from build123d import *

# Parameters (mm, degrees)
SKETCH1_R           = 25.4
BOSS_EXTRUDE1_DEPTH = 50
SKETCH2_W           = 8
SKETCH2_H           = 56.617696499
CUT_EXTRUDE1_DEPTH  = 30
SKETCH3_R           = 12.7
CUT_EXTRUDE2_DEPTH  = 35
SKETCH4_R           = 12.7
BOSS_EXTRUDE2_DEPTH = 50
BOSS_EXTRUDE3_START = -50
SKETCH5_R           = 12.7
BOSS_EXTRUDE3_DEPTH = 50


with BuildPart() as part:
    # Sketch1 → Boss-Extrude1 (new body)
    with BuildSketch(Plane.XY):
        Circle(SKETCH1_R)
    extrude(amount=BOSS_EXTRUDE1_DEPTH)

    # Sketch2 → Cut-Extrude1 (cut)
    with BuildSketch(Plane.XY.offset(50)):
        with Locations((0, -1.452503267)):
            Rectangle(SKETCH2_W, SKETCH2_H)
    extrude(amount=-CUT_EXTRUDE1_DEPTH, mode=Mode.SUBTRACT)

    # Sketch3 → Cut-Extrude2 (cut, symmetric)
    with BuildSketch(Plane.ZY.offset(-4)):
        with Locations(Location((31.954368174, 0, 0), (0, 0, 270))):
            Circle(SKETCH3_R)
    extrude(amount=CUT_EXTRUDE2_DEPTH, both=True, mode=Mode.SUBTRACT)

    # Mirror1: part across plane


with BuildPart() as part_1:
    add(part.part)
    add(part.part.mirror(Plane.XY))

    # Sketch4 → Boss-Extrude2 (add)
    with BuildSketch(Plane.ZY.offset(-4)):
        with Locations(Location((-32.054446032, 0, 0), (0, 0, 270))):
            Circle(SKETCH4_R)
    extrude(amount=-BOSS_EXTRUDE2_DEPTH)

    # Sketch5 → Boss-Extrude3 (add)
    with BuildSketch(Plane(origin=(-4, 0, 0), x_dir=(0, 0, -1), z_dir=(1, 0, 0)).offset(BOSS_EXTRUDE3_START)):
        with Locations(Location((32.054446032, 0, 0), (0, 0, 270))):
            Circle(SKETCH5_R)
    extrude(amount=BOSS_EXTRUDE3_DEPTH)


solid = part_1.part
Geometry: final body of the model. Coordinates: model frame, mm. A direction names the side the tool comes from. Round coordinates to 2 decimals unless told otherwise and drop trailing zeros. Loops run counter-clockwise (first coordinate to the right, second up) from the corner with the lowest first, then second, coordinate; pieces in that order, holes last. Notation, with made-up numbers: (69.5, 34.25) -> (84.5, 34.25) arc R11 cw to (84.5, 53.25) -> close; hole circle Ø8 at (42, -25). An arc over 180 degrees is marked (long way). One line per question, with ' | ' between items. Start each with the question number.
1. Line query: line 1 along X through (y, z) = (7, -42); line 2 along X through (y, z) = (9.5, -43); line 3 along Y through (x, z) = (4, 7.5). Output: solid intervals per line, ascending. Write a range as [from, to].
2. Section D-D on x = 12. Output: boundary loops of the cut face in (y, z), and give its area (3 significant figures).
3. Section B-B on x = 0. Output: boundary loops of the cut face in (y, z).
4. Contact query for flat-ended pins moving along their axis: pin 1 (12 mm diameter, centred on y = -0.5, z = -4.5, fed in from -X); pin 2 (2.5 mm diameter, centred on x = 1, y = -9.5, fed in from -Z); pin 3 (5 mm diameter, centred on x = -42, z = -23.5, fed in from -Y). Output: stop coordinate, or through.
5. Section A-A on y = 0. Output: boundary loops of the cut face in (x, z).
6. Section C-C on z = 28. Output: boundary loops of the cut face in (x, y).
7. Mould query, pull axis Z, two halves, no side actions, for faces 1 (the face through (-0.356, 2.753, 19.556)), 2 (the face through (12, 0, -50)), 3 (the face through (-4, 0, 45)). Classes: pulls with the +Z half, pulls with the -Z half, needs draft (parallel to the pull), parting line crosses it, or undercut.
8. Set-up query: faces 4 (the face through (0, -15, -20)), 5 (the face through (0, 15, 20)), 6 (the face through (-12, 0, -50)). Return all of +Z, -Z, +X, -X, +Y, -Y with unobstructed straight access to the full face (end or side cutting, diameter ignored); none if empty.
Returned:
1) line 1: x = [-54, -4], [4, 54] | line 2: x = [-23.56, -4], [4, 23.56] | line 3: y = [-25.08, 25.08]
2) outline: (-22.39, -50) -> (22.39, -50) -> (22.39, 50) -> (-22.39, 50) -> close; hole (-12.7, -32) arc R12.7 cw to (12.7, -32) arc R12.7 ccw (long way) to start; hole circle Ø25.4 at (0, 31.95) | area: 3,970 mm2
3) outline: (-25.4, -20) -> (-4.29, -20) arc R12.7 cw to (4.29, -20) -> (25.4, -20) -> (25.4, 20) -> (4.29, 20) arc R12.7 cw to (-4.29, 20) -> (-25.4, 20) -> close
4) pin 1: stops at x = -25.4 | pin 2: stops at z = -20 | pin 3: stops at y = -11.16
5) outline: (-54, -44.75) -> (-25.4, -44.75) -> (-25.4, -50) -> (-4, -50) -> (-4, -19.35) -> (-54, -19.35) -> close; (-25.4, -19.25) -> (25.4, -19.25) -> (25.4, 19.25) -> (-25.4, 19.25) -> close; (-25.4, 44.65) -> (-4, 44.65) -> (-4, 50) -> (-25.4, 50) -> close; (4, -50) -> (25.4, -50) -> (25.4, -44.75) -> (54, -44.75) -> (54, -19.35) -> (4, -19.35) -> close; (4, 44.65) -> (25.4, 44.65) -> (25.4, 50) -> (4, 50) -> close
6) outline: (-22.35, -12.07) arc R25.4 ccw to (-4, -25.08) -> (-4, -12.07) -> close; (-22.35, 12.07) -> (-4, 12.07) -> (-4, 25.08) arc R25.4 ccw to start; (4, -25.08) arc R25.4 ccw to (22.35, -12.07) -> (4, -12.07) -> close; (4, 12.07) -> (22.35, 12.07) arc R25.4 ccw to (4, 25.08) -> close
7) face 1: undercut | face 2: pulls with the -Z half | face 3: needs draft
8) face 4: -Z, +Y, -Y | face 5: +Z, +Y, -Y | face 6: -Z, +X, -X, +Y, -Y
